Job drawing, mm, ordinate dimensions from the low corner. One solid piece. Coordinates: 2 decimals unless noted, no trailing zeros. Order: outer loops, then holes, each group sorted by start corner. A loop starts at its lowest first (then second) coordinate and runs counter-clockwise, first axis right, second up. Notation, with made-up numbers: (-34.75, 31) - (-25.75, 31) arc R24 ccw to (-25.75, 45) - close; hole circle Ø3 at (49, 10.25). An arc over 180 degrees is marked (long way). Use a Markdown table: item, result. Add a question column.
1) Saw through at C-C on z = 0.5. Count the separate pieces of the cut face and the enclosed holes in it, then the cut area to 3 significant figures.
2) Wall check: L1, parallel to Y at x = 31.75, z = 2.45; L2, parallel to X at y = 13.5, z = 0.95; L3, parallel to X at y = 11, z = 2.45. Give the ranges that are in metal, low to high. Write a range as [from, to].
3) Saw through at A-A on x = 31.75. List the corners of the cut face in (y, z) (1 decimal), then the cut area to 3 significant figures.
4) Drop a flat-ended pin along its axis: P1, Ø6.5, axis at x = 6.35, y = 12.7, coming from the +Z side (3 decimals). Give the stop position or say it passes through.
5) Saw through at B-B on y = 12.7. List the corners of the cut face in (x, z) (1 decimal).
6) Two-plate mould, pull along X, no slides. Class the marked faces 1, 2, 3 and 4: +X half, -X half, draft (parallel to the pull), parting line (faces both ways), or undercut.
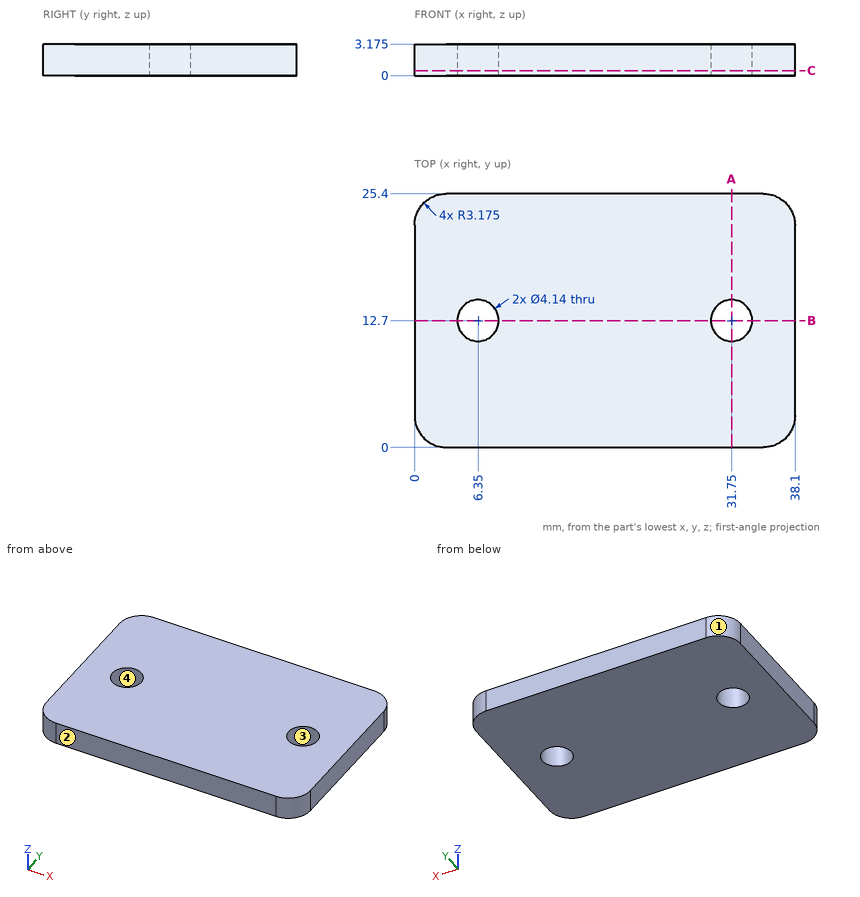
Results are:
| question | item | result |
|---|---|---|
| 1 | separate pieces | 1 |
| 1 | enclosed holes | 2 |
| 1 | area | 932 mm2 |
| 2 | L1 | [0, 10.63], [14.77, 25.4] |
| 2 | L2 | [0, 4.44], [8.26, 29.84], [33.66, 38.1] |
| 2 | L3 | [0, 5.17], [7.53, 30.57], [32.93, 38.1] |
| 3 | outline | (0, 0) - (10.6, 0) - (10.6, 3.2) - (0, 3.2) - close; (14.8, 0) - (25.4, 0) - (25.4, 3.2) - (14.8, 3.2) - close |
| 3 | area | 67.5 mm2 |
| 4 | P1 | z = 3.175 |
| 5 | outline | (0, 0) - (4.3, 0) - (4.3, 3.2) - (0, 3.2) - close; (8.4, 0) - (29.7, 0) - (29.7, 3.2) - (8.4, 3.2) - close; (33.8, 0) - (38.1, 0) - (38.1, 3.2) - (33.8, 3.2) - close |
| 6 | face 1 | -X half |
| 6 | face 2 | draft |
| 6 | face 3 | undercut |
| 6 | face 4 | undercut |
